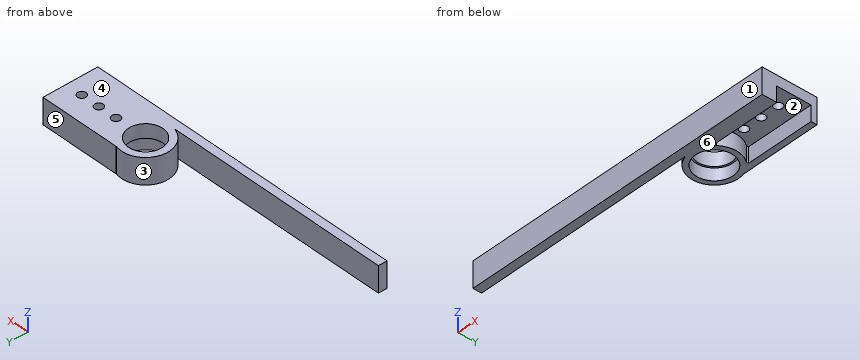
```python
from build123d import *

# Parameters (mm, degrees)
SKETCH_1_W          = 40
SKETCH_1_H          = 20
EXTRUDE_1_DEPTH     = 6
SKETCH_2_R          = 2.5
CUT_EXTRUDE_1_DEPTH = 24.151673806
EXTRUDE_START       = -15
EXTRUDE_2_OUTLINE_R = 11
EXTRUDE_2_DEPTH     = 15
EXTRUDE_START_2     = -8
SKETCH_5_R          = 11
SKETCH_5_R_2        = 10
EXTRUDE_3_DEPTH     = 8
SKETCH_10_W         = 15
SKETCH_10_H         = 5
EXTRUDE_4_DEPTH     = 500
SKETCH_11_W         = 11.491200589
SKETCH_11_H         = 5.122583395
EXTRUDE_5_DEPTH     = 15
SKETCH_13_W         = 324.526705223
SKETCH_13_H         = 235.156452348
CUT_EXTRUDE_2_DEPTH = 482.183177179
SKETCH_14_W         = 2.170521585
SKETCH_14_H         = 5
CUT_EXTRUDE_3_DEPTH = 314.479535155


# Read off the part's stored shape, not the designer's step: 凸台-拉伸2
with BuildPart() as part:
    # 草图1 → 凸台-拉伸1 (new body)
    with BuildSketch(Plane.XY):
        Rectangle(SKETCH_1_W, SKETCH_1_H)
    extrude(amount=EXTRUDE_1_DEPTH)

    # 草图2 → 切除-拉伸1 (cut, through all)
    with BuildSketch(Plane.XY.offset(6)):
        with Locations((10, 0)):
            Circle(SKETCH_2_R)
        with Locations((-1, 0)):
            Circle(SKETCH_2_R)
        with Locations((-12, 0)):
            Circle(SKETCH_2_R)
    extrude(amount=-CUT_EXTRUDE_1_DEPTH, mode=Mode.SUBTRACT)

    # 凸台-拉伸2 outline → 凸台-拉伸2 (add)
    with BuildSketch(Plane.XY.offset(6).offset(EXTRUDE_START)):
        with BuildLine():
            Line((20, 10), (20, 13.5))
            Line((20, 13.5), (-26.893967141, 13.5))
            Line((-26.893967141, 13.5), (-26.893967141, 13.384337644))
            ThreePointArc((-26.893967141, 13.384337644), (-45, 0), (-26.893967141, -13.384337644))
            Line((-26.893967141, -13.384337644), (-26.893967141, -13.5))
            Line((-26.893967141, -13.5), (20, -13.5))
            Line((20, -13.5), (20, -10))
            Line((20, -10), (-20, -10))
            Line((-20, -10), (-20, -8.660254038))
            ThreePointArc((-20, -8.660254038), (-17, 0), (-20, 8.660254038))
            Line((-20, 8.660254038), (-20, 10))
            Line((-20, 10), (20, 10))
        make_face()
        with Locations((-31, 0)):
            Circle(EXTRUDE_2_OUTLINE_R, mode=Mode.SUBTRACT)
    extrude(amount=EXTRUDE_2_DEPTH)

    # 草图5 → 凸台-拉伸3 (add)
    with BuildSketch(Plane.XY.offset(6).offset(EXTRUDE_START_2)):
        with Locations((-31, 0)):
            Circle(SKETCH_5_R)
        with Locations((-31, 0)):
            Circle(SKETCH_5_R_2, mode=Mode.SUBTRACT)
    extrude(amount=EXTRUDE_3_DEPTH)

    # 草图10 → 凸台-拉伸4 (add)
    with BuildSketch(Plane(origin=(20, 0, 0), x_dir=(0, 0, -1), z_dir=(1, 0, 0))):
        with Locations((1.5, -16)):
            Rectangle(SKETCH_10_W, SKETCH_10_H)
    extrude(amount=-EXTRUDE_4_DEPTH)

    # 草图11 → 凸台-拉伸5 (add, through all)
    with BuildSketch(Plane(origin=(0, 0, -9), x_dir=(-1, 0, 0), z_dir=(0, 0, -1))):
        with Locations((27.78271332, -13.925059853)):
            Rectangle(SKETCH_11_W, SKETCH_11_H)
    extrude(amount=-EXTRUDE_5_DEPTH)

    # 草图13 → 切除-拉伸2 (cut, through all)
    with BuildSketch(Plane.XZ.offset(18.5)):
        with Locations((-327.783817457, -102.630695063)):
            Rectangle(SKETCH_13_W, SKETCH_13_H)
    extrude(amount=-CUT_EXTRUDE_2_DEPTH, mode=Mode.SUBTRACT)

    # 草图14 → 切除-拉伸3 (cut)
    with BuildSketch(Plane.ZY.offset(480)):
        with Locations((-7.914739208, -16)):
            Rectangle(SKETCH_14_W, SKETCH_14_H)
    extrude(amount=-CUT_EXTRUDE_3_DEPTH, mode=Mode.SUBTRACT)


solid = part.part
```
Source: CAD feature listing. Evaluate the final solid. Frame: model axes, mm. Face numbers are marked on the shaded views. A direction names the side the tool comes from. Coordinates: 2 decimals unless noted, no trailing zeros. Loops run counter-clockwise (first coordinate to the right, second up) from the corner with the lowest first, then second, coordinate; pieces in that order, holes last. Notation, with made-up numbers: M 24,11 L 55,11 A30 cw 55,41 Z; hole C 30,-17.75 d5. An arc over 180 degrees is marked long. Use a Markdown table: item, result. Add a question column.
Q1. Draft query along Y for the marked faces 1, 2, 3 and 4. Return one class per face: pulls with the +Y half, pulls with the -Y half, needs draft (parallel to the pull), parting line crosses it, or undercut.
Q2. First-contact query: pin 1 (6 mm diameter, centred on x = -12, y = 0, fed in from +Z); pin 2 (12 mm diameter, centred on x = -51, y = 7.5, fed in from -Z); pin 3 (6.5 mm diameter, centred on x = 10, y = 0, fed in from -Z); pin 4 (1.5 mm diameter, centred on y = -9, z = -6.5, fed in from +X). Flat tips, straight axial feed; report the tip coordinate or a pass-through.
Q3. Section query D-D, the plane z = 2. Return loops of the section in (x, y), and give its area (3 significant figures).
Q4. Access query for the marked faces 5 and 6. Directions: +Z, -Z, +X, -X, +Y, -Y. A direction counts if a zero-diameter tool reaches every point of the face in a straight line with its end or side. Return the directions, or none.
Q5. Section query B-B, the plane x = -12. Return loops of the section in (y, z).
Q6. Material intervals for L1, parallel to Y at x = 10, z = 3; L2, parallel to Y at x = -31, z = -5; L3, parallel to Y at x = -37, z = -1, sorted ascending.
Q7. Section query A-A, the plane y = 0. Return loops of the section in (x, z), and give its area (3 significant figures).
Q8. Section query C-C, the plane z = -6.5. Return loops of the section in (x, y).
Result:
| question | item | result |
|---|---|---|
| 1 | face 1 | pulls with the -Y half |
| 1 | face 2 | undercut |
| 1 | face 3 | undercut |
| 1 | face 4 | needs draft |
| 2 | pin 1 | stops at z = 6 |
| 2 | pin 2 | passes through |
| 2 | pin 3 | stops at z = 0 |
| 2 | pin 4 | stops at x = -19.69 |
| 3 | outline | M -165.52,-18.5 L 20,-18.5 L 20,13.5 L -26.89,13.5 L -26.89,13.38 A14 ccw long -34.71,-13.5 L -165.52,-13.5 Z; hole C -31,0 d20; hole C -12,0 d5; hole C -1,0 d5; hole C 10,0 d5 |
| 3 | area | 2,240 mm2 |
| 4 | face 5 | +Z, -Z, +X, +Y |
| 4 | face 6 | -Z, +X, -X, +Y, -Y |
| 5 | outline | M -18.5,-9 L -10,-9 L -10,0 L -2.5,0 L -2.5,6 L -18.5,6 Z; M 2.5,0 L 10,0 L 10,-9 L 13.5,-9 L 13.5,6 L 2.5,6 Z |
| 6 | L1 | y = -18.5 to -2.5, 2.5 to 13.5 |
| 6 | L2 | y = -18.5 to -11, 11 to 14 |
| 6 | L3 | y = -18.5 to -13.5, -12.65 to -8, 8 to 12.65 |
| 7 | outline | M -45,-9 L -42,-9 L -42,-2 L -41,-2 L -41,6 L -45,6 Z; M -21,-2 L -20,-2 L -20,-9 L -17,-9 L -17,0 L -14.5,0 L -14.5,6 L -21,6 Z; M -9.5,0 L -3.5,0 L -3.5,6 L -9.5,6 Z; M 1.5,0 L 7.5,0 L 7.5,6 L 1.5,6 Z; M 12.5,0 L 20,0 L 20,6 L 12.5,6 Z |
| 7 | area | 238 mm2 |
| 8 | outline | M -165.52,-18.5 L 20,-18.5 L 20,-10 L -20,-10 L -20,-8.66 A14 ccw -20,8.66 L -20,10 L 20,10 L 20,13.5 L -26.89,13.5 L -26.89,13.38 A14 ccw long -34.71,-13.5 L -165.52,-13.5 Z; hole C -31,0 d22 |
